```python
from build123d import *

# Parameters (mm, degrees)
BOSS_EXTRUDE1_DEPTH           = 15
BOSS_EXTRUDE1_OTHER_WAY_DEPTH = 40
BOSS_EXTRUDE1_OTHER_WAY_TAPER = 10
BOSS_EXTRUDE2_DEPTH           = 3
BOSS_EXTRUDE3_DEPTH           = 4
BOSS_EXTRUDE3_TAPER           = 55


with BuildPart() as part:
    # Sketch1 → Boss-Extrude1 (new body)
    with BuildSketch(Plane.XY):
        with BuildLine():
            ThreePointArc((-10, -100), (0, -110), (10, -100))
            Line((10, -100), (10, 100))
            ThreePointArc((10, 100), (0, 110), (-10, 100))
            Line((-10, 100), (-10, -100))
        make_face()
    extrude(amount=BOSS_EXTRUDE1_DEPTH)

    # Sketch1 → Boss-Extrude1 other way (add)
    with BuildSketch(Plane.XY):
        with BuildLine():
            ThreePointArc((-10, -100), (0, -110), (10, -100))
            Line((10, -100), (10, 100))
            ThreePointArc((10, 100), (0, 110), (-10, 100))
            Line((-10, 100), (-10, -100))
        make_face()
    extrude(amount=-BOSS_EXTRUDE1_OTHER_WAY_DEPTH, taper=BOSS_EXTRUDE1_OTHER_WAY_TAPER)

    # Sketch2 → Boss-Extrude2 (add)
    with BuildSketch(Plane.XY.offset(15)):
        with BuildLine():
            Line((-52.5, -90), (-52.5, 90))
            ThreePointArc((-52.5, 90), (0, 142.5), (52.5, 90))
            Line((52.5, 90), (52.5, -90))
            ThreePointArc((52.5, -90), (0, -142.5), (-52.5, -90))
        make_face()
    extrude(amount=BOSS_EXTRUDE2_DEPTH)

    # Sketch3 → Boss-Extrude3 (add)
    with BuildSketch(Plane.XY.offset(18)):
        with BuildLine():
            ThreePointArc((-7, -102.5), (0, -109.5), (7, -102.5))
            Line((7, -102.5), (7, 102.5))
            ThreePointArc((7, 102.5), (0, 109.5), (-7, 102.5))
            Line((-7, 102.5), (-7, -102.5))
        make_face()
    extrude(amount=BOSS_EXTRUDE3_DEPTH, taper=BOSS_EXTRUDE3_TAPER)


solid = part.part
```
Model file for the job. Use its own axes, mm. A direction names the side the tool comes from. Round coordinates to 2 decimals unless told otherwise and drop trailing zeros. Write each loop counter-clockwise with the first axis right and the second up, starting at its lowest first coordinate (ties: lowest second). Pieces come first, ordered by that corner, then holes. Notation, with made-up numbers: (-28.5, 14.5) - (-15.5, 14.5) arc R32 ccw to (-15.5, 44.5) - close; hole circle Ø4 at (69, 14). An arc over 180 degrees is marked (long way). Use CSV: the item, a comma, the result in double quotes. Start each with the question number.
Item 1: Pin check, flat tips, straight feed: P1, Ø5, axis at y = 79.5, z = -27.5, coming from the -X side; P2, Ø8, axis at y = -64.5, z = -25.5, coming from the -X side; P3, Ø3, axis at x = 16, y = -46, coming from the -Z side; P4, Ø16.5, axis at y = 22, z = 10, coming from the -X side. Stop position of each tip, or through.
Item 2: Drill centre lines: L1, parallel to Y at x = -0.5, z = 14; L2, parallel to Z at x = -45, y = 46; L3, parallel to X at y = -15, z = 4.5. Where is each one in solid material? Low to high. Write a range as [from, to].
Item 3: Tool access for faces 1 (the face through (10, -1, 7)), 2 (the face through (-10, 1, 7)), 3 (the face through (0, -110, 7)): list every direction of +Z, -Z, +X, -X, +Y, -Y with a clear straight run to the whole face (end or side of a thin tool).
Item 4: Band-saw the part on B-B (z = 5.5). Write the cut outline in (x, y), and give its area (3 significant figures).
Item 5: Band-saw the part on A-A (y = 41.5). Write the cut outline in (x, z), and give its area (3 significant figures).
Item 6: Band-saw the part on D-D (y = 97.5). Write the cut outline in (x, z), and give its area (3 significant figures).
Item 7: Band-saw the part on C-C (x = -41). Write the cut outline in (y, z).
Checked values:
1,P1,"stops at x = -5.59"
1,P2,"stops at x = -6.21"
1,P3,"stops at z = 15"
1,P4,"stops at x = -52.5"
2,L1,"y = [-109.99, 109.99]"
2,L2,"z = [15, 18]"
2,L3,"x = [-10, 10]"
3,face 1,"-Z, +X, +Y, -Y"
3,face 2,"-Z, -X, +Y, -Y"
3,face 3,"-Z, -Y"
4,outline,"(-10, -100) arc R10 ccw to (10, -100) - (10, 100) arc R10 ccw to (-10, 100) - close"
4,area,"4,310 mm²"
5,outline,"(-52.5, 15) - (-10, 15) - (-10, 0) - (-2.95, -40) - (2.95, -40) - (10, 0) - (10, 15) - (52.5, 15) - (52.5, 18) - (7, 18) - (1.29, 22) - (-1.29, 22) - (-7, 18) - (-52.5, 18) - close"
5,area,"1,170 mm²"
6,outline,"(-51.96, 15) - (-10, 15) - (-10, 0) - (-2.95, -40) - (2.95, -40) - (10, 0) - (10, 15) - (51.96, 15) - (51.96, 18) - (7, 18) - (1.29, 22) - (-1.29, 22) - (-7, 18) - (-51.96, 18) - close"
6,area,"1,160 mm²"
7,outline,"(-122.79, 15) - (122.79, 15) - (122.79, 18) - (-122.79, 18) - close"
